from build123d import *

# Parameters (mm, degrees)
F0_W     = 25
F0_H     = 75
F1_DEPTH = 120
F2_R     = 1.525
F3_DEPTH = 1.5
F5_DEPTH = 120.001
F6_R     = 1.5
F7_DEPTH = 1.5


with BuildPart() as f1:
    # F0 (on Top) → F1 (new body)
    with BuildSketch(Plane.XY):
        Rectangle(F0_W, F0_H)
    extrude(amount=F1_DEPTH)

    # F2 (on face) → F3 (join)
    with BuildSketch(Plane.YZ.offset(12.5)):
        with Locations((-30.615, 110)):
            Circle(F2_R)
        with Locations((-30.615, 102)):
            Circle(F2_R)
        with Locations((-30.615, 94)):
            Circle(F2_R)
        with Locations((-30.615, 86)):
            Circle(F2_R)
        with Locations((-30.615, 78)):
            Circle(F2_R)
        with Locations((-30.615, 70)):
            Circle(F2_R)
        with Locations((-30.615, 62)):
            Circle(F2_R)
        with Locations((-30.615, 54)):
            Circle(F2_R)
        with Locations((-30.615, 46)):
            Circle(F2_R)
        with Locations((-30.615, 30)):
            Circle(F2_R)
        with Locations((-30.615, 38)):
            Circle(F2_R)
        with Locations((-30.615, 22)):
            Circle(F2_R)
        with Locations((-30.615, 14)):
            Circle(F2_R)
        with Locations((30.615, 110)):
            Circle(F2_R)
        with Locations((30.615, 102)):
            Circle(F2_R)
        with Locations((30.615, 94)):
            Circle(F2_R)
        with Locations((30.615, 86)):
            Circle(F2_R)
        with Locations((30.615, 78)):
            Circle(F2_R)
        with Locations((30.615, 70)):
            Circle(F2_R)
        with Locations((30.615, 62)):
            Circle(F2_R)
        with Locations((30.615, 54)):
            Circle(F2_R)
        with Locations((30.615, 46)):
            Circle(F2_R)
        with Locations((30.615, 38)):
            Circle(F2_R)
        with Locations((30.615, 30)):
            Circle(F2_R)
        with Locations((30.615, 22)):
            Circle(F2_R)
        with Locations((30.615, 14)):
            Circle(F2_R)
    extrude(amount=F3_DEPTH)

    # F4 (on face) → F5 (cut, through all)
    with BuildSketch(Plane.XY.offset(120)):
        with BuildLine():
            ThreePointArc((12.5, 2.645751), (5.5, 0), (12.5, -2.645751))
            Line((12.5, -2.645751), (12.5, 2.645751))
        make_face()
    extrude(amount=-F5_DEPTH, mode=Mode.SUBTRACT)

    # F6 (on face) → F7 (join)
    with BuildSketch(Plane(origin=(0, 0, 0), x_dir=(1, 0, 0), z_dir=(0, 0, -1))):
        with Locations((0, 32.5)):
            Circle(F6_R)
        with Locations((0, -32.5)):
            Circle(F6_R)
    extrude(amount=F7_DEPTH)


solid = f1.part
Verification items for the finished model (mm, model axes). A direction names the side the tool comes from. Give positions to 0.01 mm unless a question says otherwise; leave off trailing zeros. Loops run counter-clockwise (first coordinate to the right, second up) from the corner with the lowest first, then second, coordinate; pieces in that order, holes last.
1. Go/stop test with flat-tipped pins: P1, Ø8, axis at x = 3.5, y = -29, coming from the -Z side; P2, Ø3, axis at y = 1, z = 92, coming from the +X side; P3, Ø1, axis at y = -4, z = 54, coming from the +X side; P4, Ø4, axis at x = 4.5, y = -14.5, coming from the -Z side. Record where each tip stops, or that it passes through.
Derived:
P1: stops at z = -1.5
P2: stops at x = 6.38
P3: stops at x = 12.5
P4: stops at z = 0
2. Release check for a two-part mould opening along Z. For faces 1 (the cylindrical face through (0, -31, -1)), 2 (the cylindrical face through (13.24, -29.911, 20.647)) record: +Z half, -Z half, draft (parallel to the pull), parting line (faces both ways), or undercut.
Derived:
face 1: draft
face 2: undercut
3. Cross-section at B-B on z = 22. Record the cut outline in (x, y), and give its area (3 significant figures).
Derived:
outline: (-12.5, -37.5) - (12.5, -37.5) - (12.5, -32.14) - (14, -32.14) - (14, -29.09) - (12.5, -29.09) - (12.5, -2.65) arc R4 cw (long way) to (12.5, 2.65) - (12.5, 29.09) - (14, 29.09) - (14, 32.14) - (12.5, 32.14) - (12.5, 37.5) - (-12.5, 37.5) - close
area: 1,840 mm2
4. Cross-section at A-A on x = 9.5. Record the cut outline in (y, z), and give its area (3 significant figures).
Derived:
outline: (-37.5, 0) - (-4, 0) - (-4, 120) - (-37.5, 120) - close; (4, 0) - (37.5, 0) - (37.5, 120) - (4, 120) - close
area: 8,040 mm2
5. Cross-section at D-D on z = 65. Record the cut outline in (x, y), and give its area (3 significant figures).
Derived:
outline: (-12.5, -37.5) - (12.5, -37.5) - (12.5, -2.65) arc R4 cw (long way) to (12.5, 2.65) - (12.5, 37.5) - (-12.5, 37.5) - close
area: 1,830 mm2
6. Material ranges on probe 1 along Y at (x, z) = (9.5, 94); probe 2 along Y at (x, z) = (6.5, 105.5); probe 3 along X at (y, z) = (-19, 98), recorded low to high.
Derived:
probe 1: y = -37.5 to -4, 4 to 37.5
probe 2: y = -37.5 to -2.65, 2.65 to 37.5
probe 3: x = -12.5 to 12.5
7. Cross-section at C-C on y = 21. Record the cut outline in (x, z).
Derived:
outline: (-12.5, 0) - (12.5, 0) - (12.5, 120) - (-12.5, 120) - close
8. Tool access check on faces 3 (the cylindrical face through (13.24, -29.206, 37.416)), 4 (the flat face through (14, -31, 94)). Record the directions out of +Z, -Z, +X, -X, +Y, -Y that give a thin tool (end or side, any length) a straight path to the whole face; none if there is none.
Derived:
face 3: +X
face 4: +Z, -Z, +X, +Y, -Y
